Input: part model. Units: mm. Frame: model coordinates. Coordinates: 2 decimals unless noted, no trailing zeros. Loops run counter-clockwise (first coordinate to the right, second up) from the corner with the lowest first, then second, coordinate; pieces in that order, holes last. Notation, with made-up numbers: M 82.25,1.5 L 116.25,1.5 A16 ccw 116.25,29.5 Z; hole C 39.25,70.25 d8. An arc over 180 degrees is marked long. Use a Markdown table: item, result. Add a question column.
1. Line query: L1, parallel to X at y = 2.05, z = -29; L2, parallel to Z at x = 14.5, y = 3.35; L3, parallel to Z at x = 19, y = 1.9. Output: solid intervals per line, ascending. Write a range as [from, to].
2. Section A-A on x = 5. Output: boundary loops of the cut face in (y, z), then the cut area to 3 significant figures.
3. Draft query along X for faces 1 (the flat face through (26.247, 2.465, -14.215)), 2 (the cylindrical face through (26.818, 2.465, -31.627)), 3 (the flat face through (3.987, 2.465, -13.808)). Return one class per face: +X half, -X half, draft (parallel to the pull), parting line (faces both ways), or undercut.
4. Section B-B on y = 3.55. Output: boundary loops of the cut face in (x, z), then the cut area to 3 significant figures.
```python
from build123d import *

# Parameters (mm, degrees)
SKETCH1_R             = 2.5
BOSS_EXTRUDE1_DEPTH   = 5
F_3_0MM_DOWEL_HOLE3_D = 3


with BuildPart() as part:
    # Sketch1 → Boss-Extrude1 (new body)
    with BuildSketch(Plane(origin=(0, 0, 0), x_dir=(1, 0, 0), z_dir=(0, 1, 0))):
        with BuildLine():
            Line((7.707562498, -0.503207604), (0.160848404, 28.52631677))
            ThreePointArc((0.160848404, 28.52631677), (0.040375116, 29.15020566), (0, 29.784335781))
            Line((0, 29.784335781), (0, 120))
            ThreePointArc((0, 120), (15.064339362, 135.064339362), (30.128678723, 120))
            Line((30.128678723, 120), (30.128678723, 29.784335781))
            ThreePointArc((30.128678723, 29.784335781), (30.088303607, 29.15020566), (29.967830319, 28.52631677))
            Line((29.967830319, 28.52631677), (22.421116226, -0.503207604))
            Line((22.421116226, -0.503207604), (7.707562498, -0.503207604))
        make_face()
        with Locations(Location((5, 29.784335781, 0), (0, 0, 270))):
            Circle(SKETCH1_R, mode=Mode.SUBTRACT)
        with Locations(Location((25.128678723, 29.784335781, 0), (0, 0, 270))):
            Circle(SKETCH1_R, mode=Mode.SUBTRACT)
        with Locations(Location((25.128678723, 86.185297163, 0), (0, 0, 270))):
            Circle(SKETCH1_R, mode=Mode.SUBTRACT)
        with Locations(Location((5, 86.185297163, 0), (0, 0, 270))):
            Circle(SKETCH1_R, mode=Mode.SUBTRACT)
    extrude(amount=BOSS_EXTRUDE1_DEPTH)

    # Ø3.0mm Dowel Hole3 (through all)
    with Locations(Plane(origin=(18.290450711, 5, -7.860888975), x_dir=(0, 0, 1), z_dir=(0, 1, 0))):
        with Locations((0, 0)):
            Hole(F_3_0MM_DOWEL_HOLE3_D / 2)


solid = part.part
```
Answers below:
| question | item | result |
|---|---|---|
| 1 | L1 | x = [0.06, 2.63], [7.37, 22.75], [27.5, 30.07] |
| 1 | L2 | z = [-135.05, 0.5] |
| 1 | L3 | z = [-134.54, -9.18], [-6.54, 0.5] |
| 2 | outline | M 0,-131.21 L 5,-131.21 L 5,-88.69 L 0,-88.69 Z; M 0,-83.69 L 5,-83.69 L 5,-32.28 L 0,-32.28 Z; M 0,-27.28 L 5,-27.28 L 5,-9.91 L 0,-9.91 Z |
| 2 | area | 556 mm² |
| 3 | face 1 | +X half |
| 3 | face 2 | undercut |
| 3 | face 3 | -X half |
| 4 | outline | M 0,-120 A15.06 ccw 30.13,-120 L 30.13,-29.78 A5 ccw 29.97,-28.53 L 22.42,0.5 L 7.71,0.5 L 0.16,-28.53 A5 ccw 0,-29.78 Z; hole C 5,-86.19 d5; hole C 5,-29.78 d5; hole C 18.29,-7.86 d3; hole C 25.13,-86.19 d5; hole C 25.13,-29.78 d5 |
| 4 | area | 3,670 mm² |
